```python
from build123d import *

# Parameters (mm, degrees)
ESQUISSE15_R        = 1.5
BOSS_EXTRU_15_DEPTH = 3


with BuildPart() as part:
    # Esquisse15 → Boss.-Extru.15 (new body)
    with BuildSketch(Plane.XY):
        with BuildLine():
            Line((210.81212736, -15.397544228), (85.81212736, -15.397544228))
            ThreePointArc((85.81212736, -15.397544228), (78.741059548, -18.326476416), (75.81212736, -25.397544228))
            Line((75.81212736, -25.397544228), (75.81212736, -100.397544228))
            ThreePointArc((75.81212736, -100.397544228), (78.741059548, -107.468612039), (85.81212736, -110.397544228))
            Line((85.81212736, -110.397544228), (210.81212736, -110.397544228))
            ThreePointArc((210.81212736, -110.397544228), (217.883195172, -107.468612039), (220.81212736, -100.397544228))
            Line((220.81212736, -100.397544228), (220.81212736, -25.397544228))
            ThreePointArc((220.81212736, -25.397544228), (217.883195172, -18.326476416), (210.81212736, -15.397544228))
        make_face()
        with Locations((156.837999603, -85.008074041)):
            Circle(ESQUISSE15_R, mode=Mode.SUBTRACT)
        with Locations((156.837999603, -41.004819048)):
            Circle(ESQUISSE15_R, mode=Mode.SUBTRACT)
        with Locations((200.841254596, -41.004819048)):
            Circle(ESQUISSE15_R, mode=Mode.SUBTRACT)
        with Locations((200.841254596, -85.008074041)):
            Circle(ESQUISSE15_R, mode=Mode.SUBTRACT)
        with Locations((86.484439521, -42.744244907)):
            Circle(ESQUISSE15_R, mode=Mode.SUBTRACT)
        with Locations((134.704025572, -44.113620634)):
            Circle(ESQUISSE15_R, mode=Mode.SUBTRACT)
        with Locations((119.499920391, -94.814244907)):
            Circle(ESQUISSE15_R, mode=Mode.SUBTRACT)
        with Locations((91.564439521, -94.814244907)):
            Circle(ESQUISSE15_R, mode=Mode.SUBTRACT)
        with BuildLine():
            Line((180.960947443, -29.772427829), (212.073645815, -60.885126201))
            ThreePointArc((212.073645815, -60.885126201), (212.952325471, -63.006446545), (212.073645815, -65.127766888))
            Line((212.073645815, -65.127766888), (180.960947443, -96.24046526))
            ThreePointArc((180.960947443, -96.24046526), (178.839627099, -97.119144917), (176.718306756, -96.24046526))
            Line((176.718306756, -96.24046526), (145.605608383, -65.127766888))
            ThreePointArc((145.605608383, -65.127766888), (144.726928727, -63.006446545), (145.605608383, -60.885126201))
            Line((145.605608383, -60.885126201), (176.718306756, -29.772427829))
            ThreePointArc((176.718306756, -29.772427829), (178.839627099, -28.893748172), (180.960947443, -29.772427829))
        make_face(mode=Mode.SUBTRACT)
    extrude(amount=BOSS_EXTRU_15_DEPTH)


solid = part.part
```
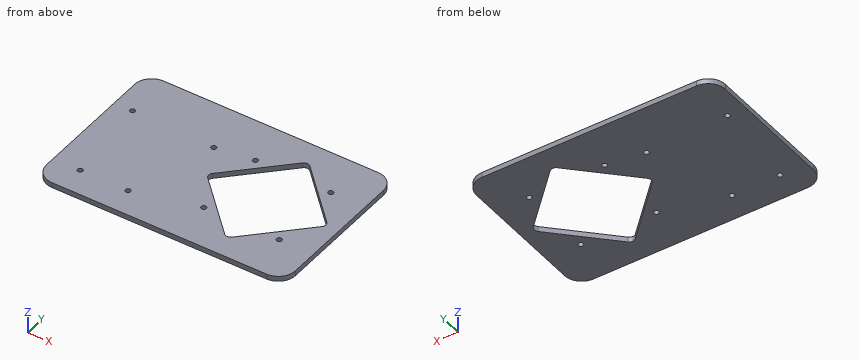
Verification items for the finished model (mm, model axes). Give positions to 0.01 mm unless a question says otherwise; leave off trailing zeros. Loops run counter-clockwise (first coordinate to the right, second up) from the corner with the lowest first, then second, coordinate; pieces in that order, holes last. Notation, with made-up numbers: M -20,83.25 L 5,83.25 A25 ccw 5,98.25 Z; hole C 33,28 d6. An arc over 180 degrees is marked long. Return JSON: item names as keys, results as strings.
1) Material ranges on L1, parallel to X at y = -41.5, z = 1.7; L2, parallel to X at y = -44, z = 1.9; L3, parallel to X at y = -84.5, z = 0.3, recorded low to high. Write a range as [from, to].
Findings:
{"L1": "x = [75.81, 85.65], [87.32, 155.42], [158.25, 164.99], [192.69, 199.43], [202.26, 220.81]", "L2": "x = [75.81, 85.66], [87.3, 133.21], [136.2, 162.49], [195.19, 220.81]", "L3": "x = [75.81, 155.43], [158.25, 164.98], [192.7, 199.43], [202.25, 220.81]"}
2) Section check A-A, the plane y = -56.5. Enter the section's corners in (x, z).
Findings:
{"outline": "M 75.81,0 L 149.99,0 L 149.99,3 L 75.81,3 Z; M 207.69,0 L 220.81,0 L 220.81,3 L 207.69,3 Z"}
3) Section check B-B, the plane x = 190. Enter the section's corners in (y, z), and give its area (3 significant figures).
Findings:
{"outline": "M -110.4,0 L -87.2,0 L -87.2,3 L -110.4,3 Z; M -38.81,0 L -15.4,0 L -15.4,3 L -38.81,3 Z", "area": "140 mm2"}
4) Section check C-C, the plane z = 2.25. Count the separate pieces of the cut face and the enclosed holes in it, and give its area (3 significant figures).
Findings:
{"separate pieces": "1", "enclosed holes": "9", "area": "11,100 mm2"}
5) Gauge pin test, flat end, axial feed: P1, Ø5, axis at x = 119.5, y = -94.81, coming from the -Z side. Record the tip position at first contact, or that the pin passes through.
Findings:
{"P1": "stops at z = 0"}
